Part model, mm, in its own coordinate system. A direction names the side the tool comes from. Round coordinates to 2 decimals unless told otherwise and drop trailing zeros. Write each loop counter-clockwise with the first axis right and the second up, starting at its lowest first coordinate (ties: lowest second). Pieces come first, ordered by that corner, then holes. Notation, with made-up numbers: M 79.25,83 L 123.25,83 A18 ccw 123.25,107 Z; hole C -15,62 d6. An arc over 180 degrees is marked long. One line per question, with ' | ' between items. Start each with the question number.
1) Tool access for faces 1 (the face through (-1, 76.7, 2)), 2 (the face through (-1, -13.493, 27)), 3 (the face through (0, -29, 16)): list every direction of +Z, -Z, +X, -X, +Y, -Y with a clear straight run to the whole face (end or side of a thin tool).
2) Drop flat-ended pins along their axis: pin 1 Ø21.5 at (y, z) = (-25, 29.5) entering from +X; pin 2 Ø2.5 at (x, z) = (-1.5, 30.5) entering from +Y; pin 3 Ø1.5 at (x, y) = (-1, -9.5) entering from +Z. Give the stop position or say it passes through.
3) Saw through at D-D (z = 3). List the corners of the cut face in (x, y).
4) Saw through at A-A (z = 19). List the corners of the cut face in (x, y), plus the area to 3 significant figures.
5) Wall check: probe 1 along X at (y, z) = (-27.5, 27.5); probe 2 along X at (y, z) = (-70, 5.5); probe 3 along Z at (x, y) = (-2.15, 65). Give the ranges that are in metal, low to high. Write a range as [from, to].
6) Saw through at C-C (y = -37.5). List the corners of the cut face in (x, z).
7) Saw through at B-B (x = -1.65). List the corners of the cut face in (y, z), plus the area to 3 significant figures.
```python
from build123d import *

# Parameters (mm, degrees)
F1_DEPTH = 11.9
F3_DEPTH = 31
F4_SIZE2 = 80.0103661193
F4_SIZE  = 7


with BuildPart() as f1:
    # F0 (on Top) → F1 (new body)
    with BuildSketch(Plane.XY):
        with BuildLine():
            Line((0, 76.7002296448), (-3, 76.7002296448))
            Line((-3, 76.7002296448), (-3, -68.2997703552))
            ThreePointArc((-3, -68.2997703552), (-1.6386286937, -74.0342530307), (2.1549561061, -78.5449445248))
            Line((2.1549561061, -78.5449445248), (2.1549561061, -74.430949986))
            ThreePointArc((2.1549561061, -74.430949986), (0.554422627, -71.5492010547), (0, -68.2997703552))
            Line((0, -68.2997703552), (0, 76.7002296448))
        make_face()
    extrude(amount=F1_DEPTH)

    # F2 (on face) → F3 (join)
    with BuildSketch(Plane.XY.offset(11.9)):
        with BuildLine():
            Line((0, -13.4931067005), (-3, -13.4931067005))
            Line((-3, -13.4931067005), (-3, -68.2997703552))
            ThreePointArc((-3, -68.2997703552), (-1.6386286937, -74.0342530307), (2.1549561061, -78.5449445248))
            Line((2.1549561061, -78.5449445248), (2.1549561061, -74.430949986))
            ThreePointArc((2.1549561061, -74.430949986), (0.554422627, -71.5492010547), (0, -68.2997703552))
            Line((0, -68.2997703552), (0, -13.4931067005))
        make_face()
    extrude(amount=F3_DEPTH)

    # F4
    f4_edges = [f1.edges().sort_by_distance(p)[0] for p in [
        (-1.5, 76.70023, 11.9),
    ]]
    f4_side = f1.faces().sort_by_distance((-1.5, 76.70023, 5.95))[0]
    chamfer(f4_edges, length=F4_SIZE, length2=F4_SIZE2, reference=f4_side)


solid = f1.part
```
Answer key:
1) face 1: +Z, -Z, +X, -X, +Y | face 2: +Z, +X, -X, +Y | face 3: +Z, -Z, +X, +Y
2) pin 1: stops at x = 0 | pin 2: stops at y = -13.49 | pin 3: stops at z = 11.9
3) outline: M -3,-68.3 A12.76 ccw 2.15,-78.54 L 2.15,-74.43 A9.8 cw 0,-68.3 L 0,76.7 L -3,76.7 Z
4) outline: M -3,-68.3 A12.76 ccw 2.15,-78.54 L 2.15,-74.43 A9.8 cw 0,-68.3 L 0,-13.49 L -3,-13.49 Z | area: 192 mm2
5) probe 1: x = [-3, 0] | probe 2: x = [-2.89, 0.15] | probe 3: z = [0, 5.92]
6) outline: M -3,0 L 0,0 L 0,42.9 L -3,42.9 Z
7) outline: M -74.01,0 L 76.7,0 L 76.7,4.9 L -3.31,11.9 L -13.49,11.9 L -13.49,42.9 L -74.01,42.9 Z | area: 3,390 mm2
